Autodesk Inventor part; units mm, degrees
ref_plane "YZ Plane" through (0, 0, 0) normal (1, 0, 0) x (0, 1, 0)
ref_plane "XZ Plane" through (0, 0, 0) normal (0, 1, 0) x (-1, 0, 0)
ref_plane "XY Plane" through (0, 0, 0) normal (0, 0, 1) x (1, 0, 0)
sketch "Boceto1" plane through (0, 0, 0) normal (0, 1, 0) x (-1, 0, 0)
  circle A0 centre (6.15, 17.029) radius 9
  dimension "d2" = 18
sketch "Boceto2" plane through (0, 0, 0) normal (0, 1, 0) x (-1, 0, 0)
  line L0 (6, -14) -> (-20.8468, 32.5)
  line L1 (-20.8468, 32.5) -> (32.8468, 32.5)
  line L2 (32.8468, 32.5) -> (6, -14)
  point P0 (0, 0)
  point P1 (6, 17)
extrude "Extrusión1" add sketch "Boceto2" along normal blind 5
extrude "Extrusión2" cut sketch "Boceto1" along normal blind 5
sketch "Boceto3" plane through (0, 0, 0) normal (0, -1, 0) x (1, 0, 0)
  circle A0 centre (-6.15, 17.029) radius 9
  line L0 (-12.3, 23.6) -> (0, 23.6)
  line L1 (0, 23.6) -> (0, 0)
  line L2 (0, 0) -> (-12.3, 0)
  line L3 (-12.3, 0) -> (-12.3, 23.6)
  point P0 (0, 0)
  point P1 (-6.15, 23.6)
  dimension "d7" = 12.3
  dimension "d8" = 23.6
extrude "Extrusión3" cut sketch "Boceto3" against normal blind 3.5 contours L1 A0 L3 L0 | L1 L2 L3 A0
sketch "Boceto4" plane through (0, 5, 0) normal (0, 1, 0) x (1, 0, 0)
  circle A0 centre (-6.15, -17.029) radius 9
  circle A1 centre (-6.15, -17.029) radius 11.0617
  point P0 (0, 0)
extrude "Extrusión4" add sketch "Boceto4" along normal blind 3
sketch "Boceto5" plane through (-32.8468, 0, 32.5) normal (0, 0, 1) x (1, 0, 0)
  line L0 (53.6936, 0) -> (0, 0)
  line L1 (0, 5) -> (53.6936, 5)
  line L2 (21.8468, 5) -> (31.8468, 5)
  line L3 (31.8468, 5) -> (31.8468, 0)
  line L4 (31.8468, 0) -> (21.8468, 0)
  line L5 (21.8468, 0) -> (21.8468, 5)
  point P0 (32.8468, 0)
  point P1 (26.8468, 0)
  point P2 (26.8468, 0)
  dimension "d13" = 10
extrude "Extrusión5" add sketch "Boceto5" along normal blind 50
sketch "Boceto6" plane through (-32.8468, 0, 32.5) normal (-0.8660254, 0, -0.5) x (-0.5, 0, 0.8660254)
  line L0 (-53.6936, 5) -> (0, 5)
  line L1 (-31.8468, 5) -> (-21.8468, 5)
  line L2 (-21.8468, 5) -> (-21.8468, 0)
  line L3 (-21.8468, 0) -> (-31.8468, 0)
  line L4 (-31.8468, 0) -> (-31.8468, 5)
  point P0 (-44.5692, 0)
  point P1 (-26.8468, 5)
  point P2 (-26.8468, 5)
  dimension "d16" = 10
  dimension "d17" = 5
extrude "Extrusión6" add sketch "Boceto6" along normal blind 50
sketch "Boceto7" plane through (-6, 0, -14) normal (0.8660254, 0, -0.5) x (-0.5, 0, -0.8660254)
  line L0 (0, 0) -> (-53.6936, 0)
  line L1 (-53.6936, 5) -> (0, 5)
  line L2 (-31.8468, 5) -> (-21.8468, 5)
  line L3 (-21.8468, 5) -> (-21.8468, 0)
  line L4 (-21.8468, 0) -> (-31.8468, 0)
  line L5 (-31.8468, 0) -> (-31.8468, 5)
  point P0 (-15.1244, 0)
  point P1 (-26.8468, 5)
  point P2 (-26.8468, 5)
  dimension "d20" = 10
extrude "Extrusión7" add sketch "Boceto7" along normal blind 50
chamfer "Chaflán1" distance 13.25 angle 45 1 edges at (-6, 2.5, -14)
sketch "Boceto8" plane through (0, 0, 0) normal (0, -1, 0) x (1, 0, 0)
  line L0 (9.9234, 13.5801) -> (20.8468, 32.5)
  line L1 (20.8468, 32.5) -> (-1, 32.5)
  line L2 (-11, 32.5) -> (-32.8468, 32.5)
  line L3 (-32.8468, 32.5) -> (-21.9234, 13.5801)
  line L4 (-16.9234, 4.9199) -> (-12.625, -2.5252)
  line L5 (-21.9234, 13.5801) -> (-11, 32.5)
  line L6 (-11, 32.5) -> (-31.0383, 44.0691)
  line L7 (-31.0383, 44.0691) -> (-41.9617, 25.1492)
  line L8 (-41.9617, 25.1492) -> (-21.9234, 13.5801)
  line L9 (-1, 32.5) -> (9.9234, 13.5801)
  line L10 (9.9234, 13.5801) -> (33.1734, 27.0035)
  line L11 (33.1734, 27.0035) -> (22.25, 45.9234)
  line L12 (22.25, 45.9234) -> (-1, 32.5)
extrude "Extrusión8" cut sketch "Boceto8" against normal blind 5 contours L9 L1 L0 | L5 L3 L2
sketch "Boceto9" plane through (0, 5, 0) normal (0, 1, 0) x (1, 0, 0)
  line L0 (48.2247, 20.0801) -> (53.2247, 11.4199)
  line L1 (-16.9234, -4.9199) -> (-60.2247, 20.0801)
  line L2 (-11, -32.5) -> (-11, -82.5)
  line L3 (-60.2247, 20.0801) -> (-57.6266, 18.5801)
  line L4 (-57.6266, 18.5801) -> (-62.6266, 9.9199)
  line L5 (-62.6266, 9.9199) -> (-65.2247, 11.4199)
  line L6 (-65.2247, 11.4199) -> (-60.2247, 20.0801)
  line L7 (48.2247, 20.0801) -> (53.2247, 11.4199)
  line L8 (53.2247, 11.4199) -> (50.6266, 9.9199)
  line L9 (50.6266, 9.9199) -> (45.6266, 18.5801)
  line L10 (45.6266, 18.5801) -> (48.2247, 20.0801)
  line L11 (-1, -82.5) -> (-11, -82.5)
  line L12 (-11, -82.5) -> (-11, -79.5)
  line L13 (-11, -79.5) -> (-1, -79.5)
  line L14 (-1, -79.5) -> (-1, -82.5)
  point P0 (0, 0)
  dimension "d31" = 3
  dimension "d32" = 3
extrude "Extrusión9" add sketch "Boceto9" along normal blind 2
properties part number "BaseVentosa"
Here's how the part is built. I have some questions about the finished solid (model axes, mm). A direction names the side the tool comes from. Give positions to 0.01 mm unless a question says otherwise; leave off trailing zeros. Write each loop counter-clockwise with the first axis right and the second up, starting at its lowest first coordinate (ties: lowest second). Pieces come first, ordered by that corner, then holes. Notation, with made-up numbers: M 38,35.25 L 79,35.25 A20 cw 79,53.25 Z; hole C 14,26 d3. An arc over 180 degrees is marked long. Put each result on its own line as item: value. Start each with the question number.
Item 1: Will these pins go through, and if not, where does the flat tip stop? pin 1 (4 mm diameter, centred on y = 2.5, z = 4.5, fed in from -X); pin 2 (2.5 mm diameter, centred on x = -5.5, y = 3.5, fed in from -Z); pin 3 (3 mm diameter, centred on x = -8, z = 4.5, fed in from -Y).
Item 2: I need wall thicknesses on L1, parallel to Z at x = -6.15, y = 6.25; L2, parallel to Z at x = -6.15, y = 2.75; L3, parallel to Z at x = -9, y = 6. Which ranges of each line are inside material? Lowest first, please. Write a range as from..to.
Item 3: If we section it at B-B, the plane z = 15: Write out the boundary of the cut face in (x, y).
Item 4: If we section it at C-C, the plane z = 61: Write out the boundary of the cut face in (x, y), then the cut area to 3 significant figures.
Item 5: Thinking about a two-plate mould opening in X: for faces 1 (the flat face through (4.385, 2.465, 23.172)), 2 (the flat face through (-14.804, 2.465, 1.249)), 3 (the flat face through (-6, 4, 82.5)), which applies, +X half, -X half, draft (parallel to the pull), parting line (faces both ways), or undercut?
Item 6: On a 3-axis mill with a long thin cutter (end or side, diameter ignored), from which of +Z, -Z, +X, -X, +Y, -Y can I reach the whole of each face in a straight line? I mean faces 4 (the flat face through (-60.1, 6, -14.3)), 5 (the flat face through (0, 2, 5)), 6 (the flat face through (-6, 3, -2.525)). Say none if no direction works.
Item 7: If we section it at D-D, the plane x = -20.5: Write out the boundary of the cut face in (y, z), then the cut area to 3 significant figures.
Values:
1. pin 1: x = -41.11
1. pin 2: z = -2.53
1. pin 3: y = 3.5
2. L1: 5.97..8.03, 26.03..28.09, 79.5..82.5
2. L2: -2.53..0, 26.03..82.5
2. L3: 6.34..8.49, 25.57..27.72, 79.5..82.5
3. outline: M -21.1,0 L -14.92,0 L -14.92,8 L -17.02,8 L -17.02,5 L -21.1,5 Z; M 2.62,0 L 9.1,0 L 9.1,5 L 4.72,5 L 4.72,8 L 2.62,8 Z
4. outline: M -11,0 L -1,0 L -1,5 L -11,5 Z
4. area: 50.0 mm²
5. face 1: +X half
5. face 2: undercut
5. face 3: draft
6. face 4: +Z, +Y
6. face 5: -Y
6. face 6: -Z, +Y, -Y
7. outline: M 0,2.85 L 5,2.85 L 5,16.05 L 0,16.05 Z
7. area: 66.0 mm²
